Autodesk Fusion 360 part; units mm, degrees
sketch "Sketch1" plane through (0, 0, 0) normal (0, 0, 1) x (1, 0, 0)
  line L0 (37.9069, 19.6511) -> (-12.0931, 19.6511)
  line L1 (-12.0931, 19.6511) -> (-12.0931, -15.3489)
  line L2 (-12.0931, -15.3489) -> (37.9069, -15.3489)
  line L3 (37.9069, -15.3489) -> (37.9069, 19.6511)
  dimension "d1" = 50
  dimension "d2" = 35
extrude "Extrude1" add sketch "Sketch1" along normal blind 25
shell "Shell1" thickness 2 removed faces 1 at (4.5736, 7.9845, 25)
fillet "Fillet1" radius 3 8 edges at (37.9069, -15.3489, 12.5) (37.9069, 19.6511, 12.5) (-10.0931, -13.3489, 13.5) (-12.0931, 19.6511, 12.5) (35.9069, 17.6511, 13.5) (-12.0931, -15.3489, 12.5) (-10.0931, 17.6511, 13.5) (35.9069, -13.3489, 13.5)
sketch "Sketch2" plane through (0, 0, 25) normal (0, 0, 1) x (-1, 0, 0)
  line L0 (-32.9069, 13.3489) -> (7.0931, 13.3489)
  arc A0 (10.0931, 10.3489) -> (7.0931, 13.3489) centre (7.0931, 10.3489) ccw
  line L1 (10.0931, 10.3489) -> (10.0931, -14.6511)
  arc A1 (7.0931, -17.6511) -> (10.0931, -14.6511) centre (7.0931, -14.6511) ccw
  line L2 (7.0931, -17.6511) -> (-32.9069, -17.6511)
  arc A2 (-35.9069, -14.6511) -> (-32.9069, -17.6511) centre (-32.9069, -14.6511) ccw
  line L3 (-35.9069, -14.6511) -> (-35.9069, 10.3489)
  arc A3 (-32.9069, 13.3489) -> (-35.9069, 10.3489) centre (-32.9069, 10.3489) ccw
  arc A4 (12.0931, 12.3489) -> (9.0931, 15.3489) centre (9.0931, 12.3489) ccw
  line L4 (9.0931, 15.3489) -> (-34.9069, 15.3489)
  arc A5 (-34.9069, 15.3489) -> (-37.9069, 12.3489) centre (-34.9069, 12.3489) ccw
  line L5 (-37.9069, 12.3489) -> (-37.9069, -16.6511)
  arc A6 (-37.9069, -16.6511) -> (-34.9069, -19.6511) centre (-34.9069, -16.6511) ccw
  line L6 (-34.9069, -19.6511) -> (9.0931, -19.6511)
  arc A7 (9.0931, -19.6511) -> (12.0931, -16.6511) centre (9.0931, -16.6511) ccw
  line L7 (12.0931, -16.6511) -> (12.0931, 12.3489)
  circle A8 centre (-21.6814, -1.7334) radius 3.5
  circle A9 centre (-3.3782, -1.7334) radius 3.5
  dimension "d8" = 7
  dimension "d9" = 7
extrude "Extrude2" cut sketch "Sketch2" against normal blind 60 contours A8 | A9
Here's how the part is built. I have some questions about the finished solid (model axes, mm). A direction names the side the tool comes from. Round coordinates to 2 decimals unless told otherwise and drop trailing zeros. Loops run counter-clockwise (first coordinate to the right, second up) from the corner with the lowest first, then second, coordinate; pieces in that order, holes last.
1. We'd pull the mould along Y, two halves only. Please class faces 3 (the face through (-12.093, 2, 12)), 4 (the face through (37.1, 18.7, 12.7)), 5 (the face through (-11.238, -14.447, 12.675)), 6 (the face through (35.1, 16.7, 13.7)): +Y half, -Y half, draft (parallel to the pull), parting line (faces both ways), or undercut.
Answer list:
face 3: draft
face 4: +Y half
face 5: -Y half
face 6: undercut
2. If we section it at A-A on x = 2: Write out the boundary of the cut face in (y, z), plus the area to 3 significant figures.
Answer list:
outline: (-15.35, 0) - (-1.48, 0) - (-1.48, 2) - (-13.35, 2) - (-13.35, 25) - (-15.35, 25) - close; (4.95, 0) - (19.65, 0) - (19.65, 25) - (17.65, 25) - (17.65, 2) - (4.95, 2) - close
area: 149 mm2
3. Which directions (+Z, -Z, +X, -X, +Y, -Y) give clear straight access to the entire face, cutting with the end or side of a thin tool? Please do faces 1 (the face through (-9.238, 16.749, 13.339)), 2 (the face through (13, -15.349, 12)).
Answer list:
face 1: +Z
face 2: +Z, -Z, +X, -X, -Y
4. If we section it at D-D on x = 30.5: Write out the boundary of the cut face in (y, z), plus the area to 3 significant figures.
Answer list:
outline: (-15.35, 0) - (19.65, 0) - (19.65, 25) - (17.65, 25) - (17.65, 2) - (-13.35, 2) - (-13.35, 25) - (-15.35, 25) - close
area: 162 mm2
5. If we section it at C-C on z = 6: Write out the boundary of the cut face in (x, y), plus the area to 3 significant figures.
Answer list:
outline: (-12.09, -12.35) arc R3 ccw to (-9.09, -15.35) - (34.91, -15.35) arc R3 ccw to (37.91, -12.35) - (37.91, 16.65) arc R3 ccw to (34.91, 19.65) - (-9.09, 19.65) arc R3 ccw to (-12.09, 16.65) - close; hole (-10.09, -10.35) arc R3 ccw to (-7.09, -13.35) - (32.91, -13.35) arc R3 ccw to (35.91, -10.35) - (35.91, 14.65) arc R3 ccw to (32.91, 17.65) - (-7.09, 17.65) arc R3 ccw to (-10.09, 14.65) - close
area: 324 mm2
6. If we section it at B-B on y = 7: Write out the boundary of the cut face in (x, z).
Answer list:
outline: (-12.09, 0) - (37.91, 0) - (37.91, 25) - (35.91, 25) - (35.91, 2) - (-10.09, 2) - (-10.09, 25) - (-12.09, 25) - close
7. If I drill on line 1 along Y through (x, z) = (26, 6.5); line 2 along X through (y, z) = (12.5, 14.75); line 3 along Z through (x, y) = (9, 15.5), over which ranges is the centre line in solid material (lowest first)?
Answer list:
line 1: y = -15.35 to -13.35, 17.65 to 19.65
line 2: x = -12.09 to -10.09, 35.91 to 37.91
line 3: z = 0 to 2
